```python
from build123d import *

# Parameters (mm, degrees)
BOSS_EXTRUDE1_DEPTH = 14
FILLET1_R           = 0.3
FILLET2_R           = 0.2
SKETCH2_W           = 2.1
SKETCH2_H           = 0.2
TAPPED_HOLE1_D      = 4.134


with BuildPart() as part:
    # Sketch1 → Boss-Extrude1 (new body)
    with BuildSketch(Plane(origin=(-4.5, 0, 0), x_dir=(0, 0, -1), z_dir=(1, 0, 0))):
        with BuildLine():
            Line((2.9, 0), (-2.9, 0))
            Line((-2.9, 0), (-2.9, -0.8))
            Line((-2.9, -0.8), (-4.77, -0.8))
            ThreePointArc((-4.77, -0.8), (-4.974026325, -0.923824397), (-4.958370592, -1.161971664))
            Line((-4.958370592, -1.161971664), (-2.9, -4.1))
            Line((-2.9, -4.1), (2.9, -4.1))
            Line((2.9, -4.1), (4.958370592, -1.161971664))
            ThreePointArc((4.958370592, -1.161971664), (4.974026325, -0.923824397), (4.77, -0.8))
            Line((4.77, -0.8), (2.9, -0.8))
            Line((2.9, -0.8), (2.9, 0))
        make_face()
    extrude(amount=BOSS_EXTRUDE1_DEPTH)

    # Fillet1
    fillet1_edges = [part.edges().sort_by_distance(p)[0] for p in [
        (2.5, -4.1, -2.9),
        (2.5, -4.1, 2.9),
    ]]
    fillet(fillet1_edges, radius=FILLET1_R)

    # Fillet2
    fillet2_edges = [part.edges().sort_by_distance(p)[0] for p in [
        (2.5, 0, 2.9),
        (2.5, 0, -2.9),
    ]]
    fillet(fillet2_edges, radius=FILLET2_R)

    # Sketch2 → Cut-Revolve1 (revolve, cut)
    with BuildSketch(Plane(origin=(6, 0, 0), x_dir=(0, 0, -1), z_dir=(1, 0, 0))):
        with Locations((1.05, -4)):
            Rectangle(SKETCH2_W, SKETCH2_H)
    revolve(axis=Axis((6, 1.665548573, 0), (0, -1, 0)), mode=Mode.SUBTRACT)

    # Sketch3 → Revolve1 (revolve)
    with BuildSketch(Plane(origin=(6, 0, 0), x_dir=(0, 0, -1), z_dir=(1, 0, 0))):
        with BuildLine():
            Line((1.670329309, -3.9), (0, -3.9))
            Line((0, -3.9), (0, -4.8))
            ThreePointArc((0, -4.8), (0.948683298, -4.560681686), (1.670329309, -3.9))
        make_face()
    revolve(axis=Axis((6, 0, 0), (0, -1, 0)))

    # Tapped Hole1 (through all)
    with Locations(Plane(origin=(0, 0, 0), x_dir=(1, 0, 0), z_dir=(0, 1, 0))):
        with Locations((0, 0)):
            Hole(TAPPED_HOLE1_D / 2)


solid = part.part
```
Check sheet for the modelled part. Datum: model origin and axes. Units: mm. A direction names the side the tool comes from. Give positions to 0.01 mm unless a question says otherwise; leave off trailing zeros. Write each loop counter-clockwise with the first axis right and the second up, starting at its lowest first coordinate (ties: lowest second). Pieces come first, ordered by that corner, then holes.
Item 1: Draft check along X on faces 1 (the face through (1.64, -2.08, 1.26)), 2 (the face through (2.4, -2.59, -3.96)), 3 (the face through (9.5, -2, 0)). Enter one of: released by +X, released by -X, zero draft, split by the parting line, or undercut.
Item 2: Cross-section at D-D (x = 6). Enter the section's corners in (y, z), and give its area (3 significant figures).
Item 3: Gauge pin test, flat ends, axial feed: pin 1 (1.5 mm diameter, centred on x = 1.5, z = 4, fed in from +Y); pin 2 (0.5 mm diameter, centred on x = -0.5, y = -0.5, fed in from +Z); pin 3 (5.5 mm diameter, centred on x = 0, z = 0, fed in from -Y). Record the tip position at first contact, or that the pin passes through.
Item 4: Cross-section at C-C (y = -1.65). Enter the section's corners in (x, z).
Item 5: Access from +Z, -Z, +X, -X, +Y, -Y to the whole of each face (thin tool, end or side, straight path). Record for faces 4 (the face through (2, -0.8, 4)), 5 (the face through (2, -0.8, -4)), 6 (the face through (-4.5, -2, 0)).
Item 6: Scan lines: L1, parallel to Y at x = 6.75, z = -2.5; L2, parallel to Z at x = 0, y = -2.4; L3, parallel to X at y = -3.6, z = -1.25. Record each from-to range of solid material in increasing order.
Item 7: Cross-section at A-A (x = 0). Enter the section's corners in (y, z), and give its area (3 significant figures).
Item 8: Cross-section at B-B (z = 0). Enter the section's corners in (x, y).
Report:
1. face 1: undercut
1. face 2: zero draft
1. face 3: released by +X
2. outline: (-4.1, -2.74) arc R0.3 ccw to (-3.97, -2.99) - (-1.16, -4.96) arc R0.23 ccw to (-0.8, -4.77) - (-0.8, -2.9) - (-0.2, -2.9) arc R0.2 ccw to (0, -2.7) - (0, 2.7) arc R0.2 ccw to (-0.2, 2.9) - (-0.8, 2.9) - (-0.8, 4.77) arc R0.23 ccw to (-1.16, 4.96) - (-3.97, 2.99) arc R0.3 ccw to (-4.1, 2.74) - (-4.1, 2.1) - (-3.9, 2.1) - (-3.9, 1.67) arc R2 ccw to (-3.9, -1.67) - (-3.9, -2.1) - (-4.1, -2.1) - close
2. area: 32.6 mm2
3. pin 1: stops at y = -0.8
3. pin 2: stops at z = 2.9
3. pin 3: stops at y = -4.1
4. outline: (-4.5, -4.62) - (9.5, -4.62) - (9.5, 4.62) - (-4.5, 4.62) - close; hole circle Ø4.13 at (0, 0)
5. face 4: +Z, +X, -X, +Y
5. face 5: -Z, +X, -X, +Y
5. face 6: +Z, -Z, -X, +Y, -Y
6. L1: y = -4.1 to 0
6. L2: z = -4.09 to -2.07, 2.07 to 4.09
6. L3: x = -4.5 to -1.65, 1.65 to 9.5
7. outline: (-4.1, -2.74) arc R0.3 ccw to (-3.97, -2.99) - (-1.16, -4.96) arc R0.23 ccw to (-0.8, -4.77) - (-0.8, -2.9) - (-0.2, -2.9) arc R0.2 ccw to (0, -2.7) - (0, -2.07) - (-4.1, -2.07) - close; (-4.1, 2.07) - (0, 2.07) - (0, 2.7) arc R0.2 ccw to (-0.2, 2.9) - (-0.8, 2.9) - (-0.8, 4.77) arc R0.23 ccw to (-1.16, 4.96) - (-3.97, 2.99) arc R0.3 ccw to (-4.1, 2.74) - close
7. area: 14.3 mm2
8. outline: (-4.5, -4.1) - (-2.07, -4.1) - (-2.07, 0) - (-4.5, 0) - close; (2.07, -4.1) - (3.9, -4.1) - (3.9, -3.9) - (4.33, -3.9) arc R2 ccw to (7.67, -3.9) - (8.1, -3.9) - (8.1, -4.1) - (9.5, -4.1) - (9.5, 0) - (2.07, 0) - close
